Part model, mm, in its own coordinate system. A direction names the side the tool comes from. Coordinates: 2 decimals unless noted, no trailing zeros. Order: outer loops, then holes, each group sorted by start corner. A loop starts at its lowest first (then second) coordinate and runs counter-clockwise, first axis right, second up.
1) Pin check, flat tips, straight feed: pin 1 Ø7 at (x, y) = (-24, 30.5) entering from -Z; pin 2 Ø5 at (x, y) = (-26, 31) entering from +Z; pin 3 Ø0.6 at (x, z) = (-2, 225.5) entering from +Y. Stop position of each tip, or through.
2) Cut at A-A (z = -55). List the corners of the cut face in (x, y).
3) Cut at C-C (y = 23.5). List the corners of the cut face in (x, z), and give its area (3 significant figures).
4) Tool access for faces 1 (the flat face through (0, 14, 21)), 2 (the flat face through (-20, 29.356, 21)): list every direction of +Z, -Z, +X, -X, +Y, -Y with a clear straight run to the whole face (end or side of a thin tool).
5) Cut at B-B (x = -30). List the corners of the cut face in (y, z), and give its area (3 significant figures).
6) Wall check: L1, parallel to X at y = 6, z = -31; L2, parallel to Y at x = -31.5, z = 122.5; L3, parallel to Z at x = -2.5, y = 25. Give the ranges that are in metal, low to high.
```python
from build123d import *

# Parameters (mm, degrees)
BASE_FLANGE1_DEPTH            = 4
EDGE_FLANGE1_STRIP_W          = 16.4
EDGE_FLANGE1_STRIP_H          = 4
EDGE_FLANGE1_STRIP_CUT_DEPTH  = 412.942027617
EDGE_FLANGE1_RELIEF_W         = 18.4
EDGE_FLANGE1_RELIEF_H         = 2
EDGE_FLANGE1_RELIEF_CUT_DEPTH = 4
EDGE_FLANGE1_DEPTH            = 412.942027617


# Sheet-metal steps are written as plain solids
with BuildPart() as part:
    # Sketch1 → Base-Flange1 (new body)
    with BuildSketch(Plane(origin=(0, 0, 0), x_dir=(0, 0, -1), z_dir=(1, 0, 0))):
        with BuildLine():
            Line((188.350009653, 33.355878637), (-224.592017965, 33.355878637))
            Line((-224.592017965, 33.355878637), (-236.864654255, 6.041062278))
            ThreePointArc((-236.864654255, 6.041062278), (-237.017988994, 2.32545676), (-234.563610744, -0.468333375))
            Line((-234.563610744, -0.468333375), (-232.242884183, -1.644121363))
            Line((-232.242884183, -1.644121363), (196.000875871, -1.644121363))
            Line((196.000875871, -1.644121363), (198.321602432, -0.468333375))
            ThreePointArc((198.321602432, -0.468333375), (200.775980682, 2.32545676), (200.622645942, 6.041062278))
            Line((200.622645942, 6.041062278), (188.350009653, 33.355878637))
        make_face()
    extrude(amount=-BASE_FLANGE1_DEPTH)

    # Edge-Flange1 strip (across the edge) → Edge-Flange1 strip cut (cut)
    with BuildSketch(Plane(origin=(-4, 33.355878637, 224.592017965), x_dir=(0, -1, 0), z_dir=(0, 0, -1))):
        with Locations((-4, -2)):
            Rectangle(EDGE_FLANGE1_STRIP_W, EDGE_FLANGE1_STRIP_H)
    extrude(amount=EDGE_FLANGE1_STRIP_CUT_DEPTH, mode=Mode.SUBTRACT)

    # Edge-Flange1 relief (on the sheet) → Edge-Flange1 relief cut (cut)
    with BuildSketch(Plane(origin=(-4, 29.155878637, 224.592017965), x_dir=(0, -1, 0), z_dir=(-1, 0, 0))):
        with Locations((-7.2, 1)):
            Rectangle(EDGE_FLANGE1_RELIEF_W, EDGE_FLANGE1_RELIEF_H)
        with Locations((-7.2, -413.942027617)):
            Rectangle(EDGE_FLANGE1_RELIEF_W, EDGE_FLANGE1_RELIEF_H)
    extrude(amount=-EDGE_FLANGE1_RELIEF_CUT_DEPTH, mode=Mode.SUBTRACT)

    # Edge-Flange1 section (across the edge) → Edge-Flange1 (add)
    with BuildSketch(Plane(origin=(-4, 33.355878637, 224.592017965), x_dir=(0, -1, 0), z_dir=(0, 0, -1))):
        with BuildLine():
            Line((0, 0.2), (0, 31))
            Line((0, 31), (4, 31))
            Line((4, 31), (4, 0.2))
            ThreePointArc((4, 0.2), (4.058578644, 0.058578644), (4.2, 0))
            Line((4.2, 0), (4.2, -4))
            ThreePointArc((4.2, -4), (1.230151519, -2.769848481), (0, 0.2))
        make_face()
    extrude(amount=EDGE_FLANGE1_DEPTH)


solid = part.part
```
Geometry check:
1. pin 1: stops at z = -188.35
1. pin 2: stops at z = 224.59
1. pin 3: stops at y = 27.16
2. outline: (-35, 29.36) - (-4.2, 29.36) arc R0.2 cw to (-4, 29.16) - (-4, -1.64) - (0, -1.64) - (0, 29.16) arc R4.2 ccw to (-4.2, 33.36) - (-35, 33.36) - close
3. outline: (-4, -192.78) - (0, -192.78) - (0, 229.02) - (-4, 229.02) - close
3. area: 1,690 mm2
4. face 1: +Z, -Z, +X, +Y, -Y
4. face 2: +Z, -Z, -X, -Y
5. outline: (29.36, -188.35) - (33.36, -188.35) - (33.36, 224.59) - (29.36, 224.59) - close
5. area: 1,650 mm2
6. L1: x = -4 to 0
6. L2: y = 29.36 to 33.36
6. L3: z = -192.1 to 228.35
